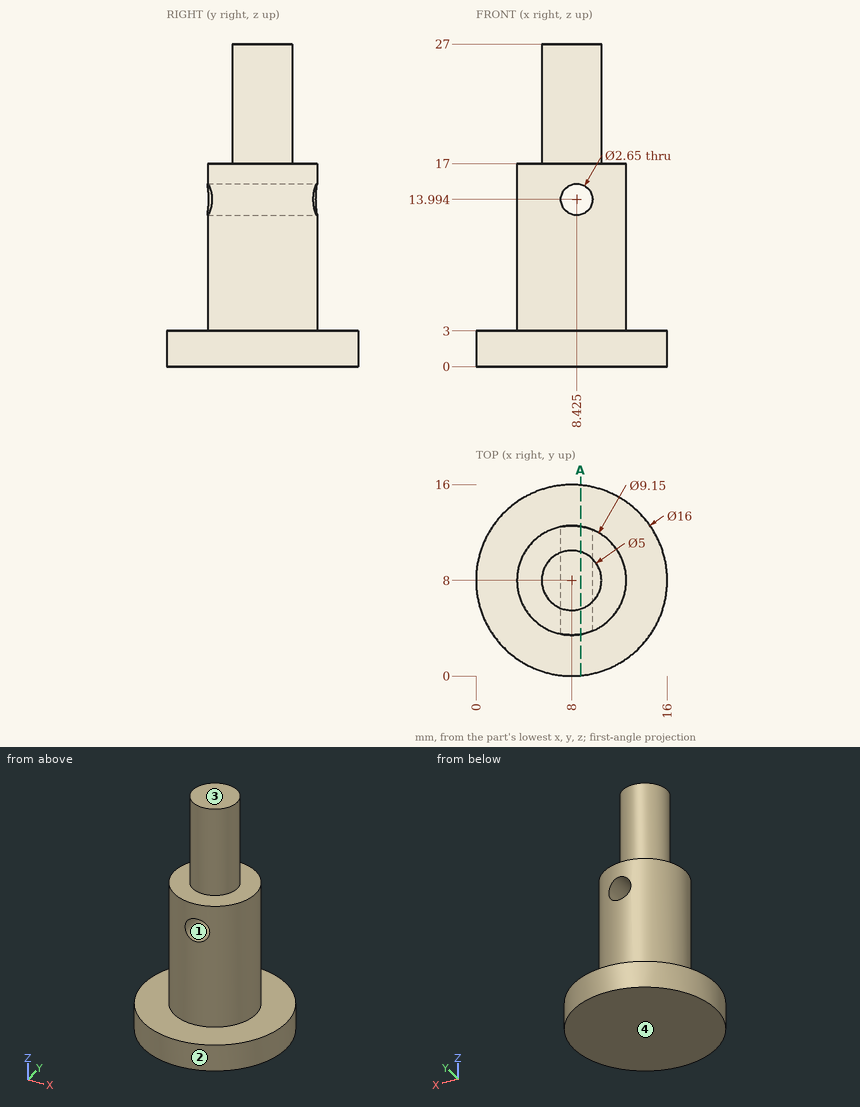
Here's the drawing with two shaded views (mm, measured from the low corner). I have some questions. Round coordinates to 2 decimals unless told otherwise and drop trailing zeros. Order: outer loops, then holes, each group sorted by start corner. A loop starts at its lowest first (then second) coordinate and runs counter-clockwise, first axis right, second up. Notation, with made-up numbers: (68.5, -10) -> (90.5, -10) arc R13 cw to (90.5, -3) -> close; hole circle Ø8 at (87, 80). An arc over 180 degrees is marked (long way). Write each question's results on one line, items separated by ' | '. Start each with the question number.
Item 1: If we section it at A-A, the plane x = 8.75: Write out the boundary of the cut face in (y, z) (1 decimal), then the cut area to 3 significant figures.
Item 2: Thinking about a two-plate mould opening in Z: for the marked faces 1, 2, 3 and 4, which applies, +Z half, -Z half, draft (parallel to the pull), parting line (faces both ways), or undercut?
Item 3: Please list where these lines run through material, in increasing order: L1, parallel to Z at x = 10.5, y = 13.5; L2, parallel to Z at x = 5.5, y = 11.25; L3, parallel to X at y = 11, z = 13.75 (1 decimal).
Item 4: Will these pins go through, and if not, where does the flat tip stop? pin 1 (1.5 mm diameter, centred on y = 7, z = 14.5, fed in from -X); pin 2 (5 mm diameter, centred on x = 10.5, z = 20.5, fed in from +Y); pin 3 (3 mm diameter, centred on x = 8.43, z = 13.99, fed in from +Y) (3 decimals); pin 4 (6 mm diameter, centred on x = 7.5, y = 11, fed in from +Z).
Results:
1) outline: (0, 0) -> (16, 0) -> (16, 3) -> (12.5, 3) -> (12.5, 12.7) -> (3.5, 12.7) -> (3.5, 3) -> (0, 3) -> close; (3.5, 15.3) -> (12.5, 15.3) -> (12.5, 17) -> (10.4, 17) -> (10.4, 27) -> (5.6, 27) -> (5.6, 17) -> (3.5, 17) -> close | area: 199 mm2
2) face 1: undercut | face 2: draft | face 3: +Z half | face 4: -Z half
3) L1: z = 0 to 3 | L2: z = 0 to 17 | L3: x = 4.5 to 7.1, 9.7 to 11.5
4) pin 1: stops at x = 3.43 | pin 2: stops at y = 10.5 | pin 3: stops at y = 12.575 | pin 4: stops at z = 27
